Part print with two shaded views. Sizes in mm from the minimum x, y, z corner. Round coordinates to 2 decimals unless told otherwise and drop trailing zeros. Write each loop counter-clockwise with the first axis right and the second up, starting at its lowest first coordinate (ties: lowest second). Pieces come first, ordered by that corner, then holes.
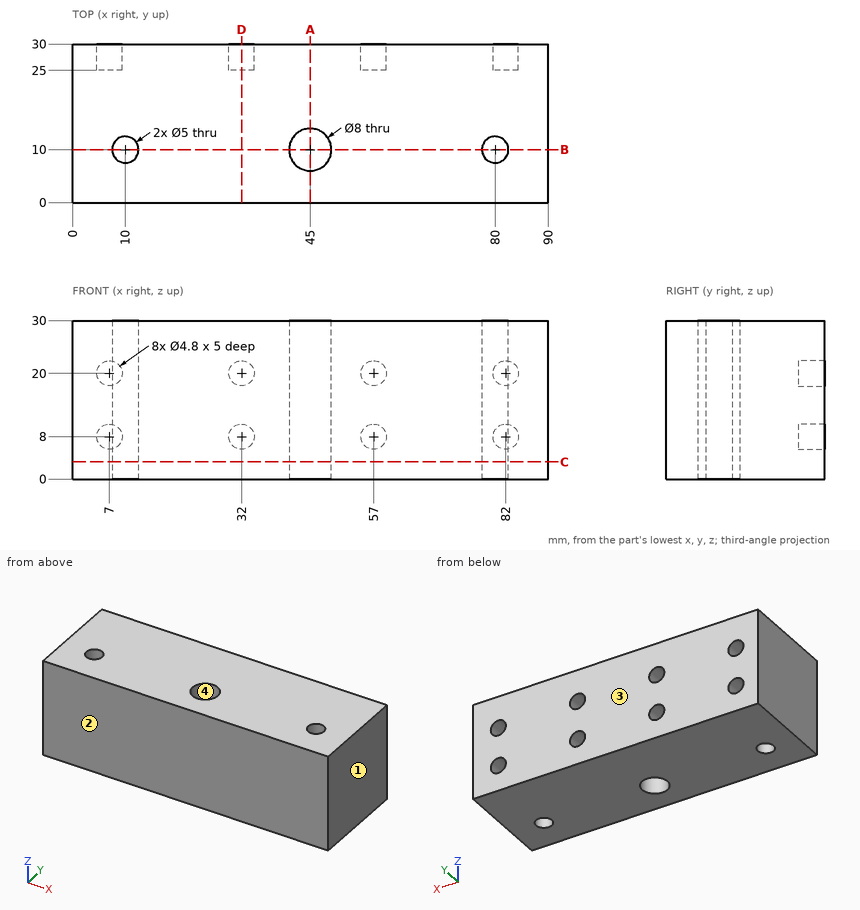
Q1. Cut at D-D on x = 32. Write the cut outline in (y, z).
Values follow:
outline: (0, 0) - (30, 0) - (30, 5.6) - (25, 5.6) - (25, 10.4) - (30, 10.4) - (30, 17.6) - (25, 17.6) - (25, 22.4) - (30, 22.4) - (30, 30) - (0, 30) - close
Q2. Drop a flat-ended pin along its axis: pin 1 (4 mm diameter, centred on x = 32, z = 8, fed in from +Y). Give the stop position or say it passes through.
Values follow:
pin 1: stops at y = 25
Q3. Cut at A-A on x = 45. Write the cut outline in (y, z), plus the area to 3 significant figures.
Values follow:
outline: (0, 0) - (6, 0) - (6, 30) - (0, 30) - close; (14, 0) - (30, 0) - (30, 30) - (14, 30) - close
area: 660 mm2
Q4. Cut at B-B on y = 10. Write the cut outline in (x, z), plus the area to 3 significant figures.
Values follow:
outline: (0, 0) - (7.5, 0) - (7.5, 30) - (0, 30) - close; (12.5, 0) - (41, 0) - (41, 30) - (12.5, 30) - close; (49, 0) - (77.5, 0) - (77.5, 30) - (49, 30) - close; (82.5, 0) - (90, 0) - (90, 30) - (82.5, 30) - close
area: 2,160 mm2
Q5. Wall check: L1, parallel to X at y = 28.8, z = 8; L2, parallel to Y at x = 10, z = 16; L3, parallel to X at y = 25.25, z = 18. Give the ranges that are in metal, low to high.
Values follow:
L1: x = 0 to 4.6, 9.4 to 29.6, 34.4 to 54.6, 59.4 to 79.6, 84.4 to 90
L2: y = 0 to 7.5, 12.5 to 30
L3: x = 0 to 5.67, 8.33 to 30.67, 33.33 to 55.67, 58.33 to 80.67, 83.33 to 90
Q6. Mould opens along Y. For the marked faces 1, 2, 3 and 4 say: +Y half, -Y half, draft (parallel to the pull), parting line (faces both ways), or undercut.
Values follow:
face 1: draft
face 2: -Y half
face 3: +Y half
face 4: undercut
Q7. Cut at C-C on z = 3.25. Write the cut outline in (x, y), plus the area to 3 significant figures.
Values follow:
outline: (0, 0) - (90, 0) - (90, 30) - (0, 30) - close; hole circle Ø5 at (10, 10); hole circle Ø8 at (45, 10); hole circle Ø5 at (80, 10)
area: 2,610 mm2
